CAD build for the part. Positions are in the model's coordinates, mm. Face numbers are marked on the shaded views. A direction names the side the tool comes from. Coordinates: 2 decimals unless noted, no trailing zeros. Order: outer loops, then holes, each group sorted by start corner. A loop starts at its lowest first (then second) coordinate and runs counter-clockwise, first axis right, second up.
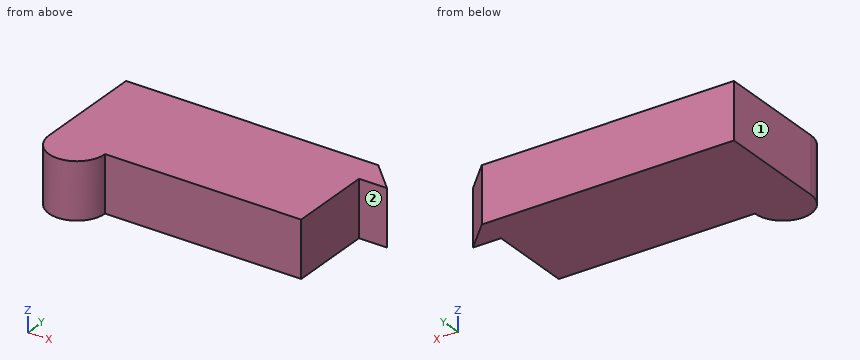
from build123d import *

# Parameters (mm, degrees)
BOSS_EXTRUDE1_DEPTH = 508


with BuildPart() as part:
    # Sketch1 → Boss-Extrude1 (new body)
    with BuildSketch(Plane.XY):
        with BuildLine():
            Line((-1664.53924545, 1529.861538462), (621.46075455, 1529.861538462))
            Line((621.46075455, 1529.861538462), (876.093987038, 1275.228305974))
            Line((876.093987038, 1275.228305974), (622.093987038, 1275.228305974))
            Line((622.093987038, 1275.228305974), (622.093987038, 513.228305974))
            Line((622.093987038, 513.228305974), (-1155.906012962, 513.228305974))
            ThreePointArc((-1155.906012962, 513.228305974), (-1410.53924545, 259.228305974), (-1664.53924545, 513.861538462))
            Line((-1664.53924545, 513.861538462), (-1664.53924545, 1529.861538462))
        make_face()
    extrude(amount=BOSS_EXTRUDE1_DEPTH)


solid = part.part
1) Slice it at B-B (x = 17). List the corners of the cut face in (y, z), plus the area to 3 significant figures.
2) Which spindle directions (+Z, -Z, +X, -X, +Y, -Y) get a long thin tool onto all of the face, cutting with end or side? Do the marked faces 1 and 2. Say none if no direction does.
3) Slice it at C-C (y = 729.5). List the corners of the cut face in (x, z).
4) Slice it at A-A (z = 201). List the corners of the cut face in (x, y), plus the area to 3 significant figures.
5) Pin check, flat tips, straight feed: P1, Ø1.5, axis at y = 388.5, z = 242, coming from the +X side; P2, Ø12, axis at y = 430, z = 322, coming from the -X side; P3, Ø4, axis at y = 1006.5, z = 424.5, coming from the +X side. Stop position of each tip, or through.
6) Drill centre lines: probe 1 along Y at (x, z) = (305.5, 99); probe 2 along Y at (x, z) = (-1423, 89); probe 3 along X at (y, z) = (801, 245). Where is each one in solid material? Low to high.
Worked out:
1. outline: (513.23, 0) - (1529.86, 0) - (1529.86, 508) - (513.23, 508) - close
1. area: 516,000 mm2
2. face 1: +Z, -Z, -X, +Y, -Y
2. face 2: +Z, -Z, +X, -Y
3. outline: (-1664.54, 0) - (622.09, 0) - (622.09, 508) - (-1664.54, 508) - close
4. outline: (-1664.54, 513.86) arc R254.32 ccw to (-1155.91, 513.23) - (622.09, 513.23) - (622.09, 1275.23) - (876.09, 1275.23) - (621.46, 1529.86) - (-1664.54, 1529.86) - close
4. area: 2,460,000 mm2
5. P1: stops at x = -1188.35
5. P2: stops at x = -1652.43
5. P3: stops at x = 622.09
6. probe 1: y = 513.23 to 1529.86
6. probe 2: y = 259.55 to 1529.86
6. probe 3: x = -1664.54 to 622.09
